Build history of the part. All positions in model axes, mm. A direction names the side the tool comes from. Give positions to 0.01 mm unless a question says otherwise; leave off trailing zeros. Order: outer loops, then holes, each group sorted by start corner. A loop starts at its lowest first (then second) coordinate and runs counter-clockwise, first axis right, second up. Notation, with made-up numbers: (81.5, -21) -> (85.5, -21) arc R21 cw to (85.5, 9) -> close; hole circle Ø3 at (18, 15). An arc over 180 degrees is marked (long way). One line per question, with ' | ' between items. Start each with the question number.
(1) Cut at A-A (y = -131). Give the cut face in (x, z) (3 decimals).
(2) Pull direction Y, two halves, no side cores. Call faces 3 (the face through (-13.858, -2.348, 10.626)), 4 (the face through (-3.172, -90.685, -24.613)), 5 (the face through (-3.172, -90.685, 24.613)), 6 (the face through (21, 0, 1)): +Y half, -Y half, draft (parallel to the pull), parting line (faces both ways), or undercut.
(3) Which spindle directions (+Z, -Z, +X, -X, +Y, -Y) get a long thin tool onto all of the face, cutting with end or side? Do faces 1 (the face through (-1, -250.825, 1)), 2 (the face through (-1.707, -48.396, -2.677)). Say none if no direction does.
(4) Drill centre lines: L1, parallel to Y at x = 0, z = 27.5 (3 decimals); L2, parallel to Y at x = -40, z = 0 (3 decimals); L3, parallel to Z at x = -0.5, y = -22. Where is each one in solid material? Low to high. Write a range as from..to.
(5) Pin check, flat tips, straight feed: pin 1 Ø10 at (x, y) = (-6, -133) entering from -Z; pin 2 Ø12 at (y, z) = (-25, 8) entering from -X; pin 3 Ø6 at (y, z) = (-137.5, -21) entering from +X; pin 4 Ø1 at (x, z) = (-27, 16) entering from +Y. Stop position of each tip, or through.
(6) Cut at B-B (y = -176). Give the cut face in (x, z), then the cut area to 3 significant figures.
from build123d import *

# Parameters (mm, degrees)
F0_R           = 49.9237
F1_DEPTH       = 250.825
F2_SIZE2       = 1.7014773719
F2_SIZE        = 6.35
F4_D           = 6.35
F4_DEPTH       = 158.75
F4_CBORE_D     = 34.925
F4_CBORE_DEPTH = 4.7625
F4_TIP         = 1.9077324654
F5_R           = 3.175
F6_DEPTH       = 49.9247
F6_DEPTH_BACK  = 49.9247
F7_R           = 3.175
F8_DEPTH       = 49.9247001
F8_DEPTH_BACK  = 49.9247001
F9_SIZE        = 1


with BuildPart() as f1:
    # F0 (on Front) → F1 (new body)
    with BuildSketch(Plane.XZ):
        Circle(F0_R)
    extrude(amount=F1_DEPTH)

    # F2
    f2_edges = [f1.edges().sort_by_distance(p)[0] for p in [
        (-49.9237, -250.825, 0),
    ]]
    f2_side = f1.faces().sort_by_distance((-49.9237, -125.4125, 0))[0]
    chamfer(f2_edges, length=F2_SIZE, length2=F2_SIZE2, reference=f2_side)

    # F4
    with Locations(Plane(origin=(0, 0, 0), x_dir=(1, 0, 0), z_dir=(0, 1, 0))):
        with Locations((0, 0)):
            CounterBoreHole(F4_D / 2, F4_CBORE_D / 2, F4_CBORE_DEPTH, depth=F4_DEPTH)
            with Locations((0, 0, -(F4_DEPTH + F4_TIP / 2))):  # 118° drill point
                Cone(0, F4_D / 2, F4_TIP, mode=Mode.SUBTRACT)

    # F5 (on Right) → F6 (cut, two sides)
    with BuildSketch(Plane.YZ) as f6_sk:
        with Locations((-160.825, 0)):
            Circle(F5_R)
    extrude(amount=-F6_DEPTH, mode=Mode.SUBTRACT)
    extrude(f6_sk.sketch, amount=F6_DEPTH_BACK, mode=Mode.SUBTRACT)

    # F7 (on Top) → F8 (cut, two sides)
    with BuildSketch(Plane.XY) as f8_sk:
        with Locations((0, -90.825)):
            Circle(F7_R)
    extrude(amount=-F8_DEPTH, mode=Mode.SUBTRACT)
    extrude(f8_sk.sketch, amount=F8_DEPTH_BACK, mode=Mode.SUBTRACT)

    # F9
    f9_edges = [f1.edges().sort_by_distance(p)[0] for p in [
        (-49.9237, 0, 0),
    ]]
    chamfer(f9_edges, length=F9_SIZE)


solid = f1.part
Result set:
1) outline: circle Ø99.847 at (0, 0); hole circle Ø6.35 at (0, 0)
2) face 3: draft | face 4: undercut | face 5: undercut | face 6: +Y half
3) face 1: +Z, -Z, +X, -X, -Y | face 2: +Y
4) L1: y = -250.825..-94, -87.65..0 | L2: y = -250.825..-164, -157.65..0 | L3: z = -49.92..-3.14, 3.14..49.92
5) pin 1: stops at z = -49.91 | pin 2: stops at x = -49.88 | pin 3: stops at x = 46.57 | pin 4: stops at y = 0
6) outline: circle Ø99.85 at (0, 0) | area: 7,830 mm2
